```python
from build123d import *

# Parameters (mm, degrees)
F0_R     = 28.446673
F1_DEPTH = 25
F2_W     = 12.863994
F2_H     = 8.371785
F3_DEPTH = 25
F5_DEPTH = 25
F6_R     = 14.342599
F7_DEPTH = 125


with BuildPart() as f1:
    # F0 (on Front) → F1 (new body)
    with BuildSketch(Plane.XZ):
        Circle(F0_R)
    extrude(amount=F1_DEPTH)

    # F2 (on Front) → F3 (cut)
    with BuildSketch(Plane.XZ):
        with Locations((-6.431997, 4.185892)):
            Rectangle(F2_W, F2_H)
    extrude(amount=F3_DEPTH, mode=Mode.SUBTRACT)

    # F4 (on Front) → F5 (cut)
    with BuildSketch(Plane.XZ):
        Polygon((13.908368, -11.549142), (9.61332, 23.327414), (2.882242, 23.327414), (6.163642, -12.263194), align=None)
    extrude(amount=F5_DEPTH, mode=Mode.SUBTRACT)

    # F6 (on Front) → F7 (join)
    with BuildSketch(Plane.XZ):
        Circle(F6_R)
    extrude(amount=-F7_DEPTH)


solid = f1.part
```
Part model, mm, in its own coordinate system. A direction names the side the tool comes from. Round coordinates to 2 decimals unless told otherwise and drop trailing zeros. Write each loop counter-clockwise with the first axis right and the second up, starting at its lowest first coordinate (ties: lowest second). Pieces come first, ordered by that corner, then holes. Notation, with made-up numbers: (26.25, -24) -> (70.25, -24) arc R35 cw to (70.25, 14) -> close; hole circle Ø11 at (9, -22.5). An arc over 180 degrees is marked (long way). Return JSON: item names as keys, results as strings. Group by question number.
Q1. Saw through at B-B on y = 57. Write the cut outline in (x, z).
Q2. Probe L1, parallel to Y at x = 10, z = 2.5; L2, parallel to Y at x = -14.5, z = -7; L3, parallel to Z at x = -16, y = -16. List the from-to ranges inside material, lowest first. Write a range as [from, to].
Q3. Saw through at A-A on z = 21. Write the cut outline in (x, y).
Q4. Pin check, flat tips, straight feed: pin 1 (1.5 mm diameter, centred on x = -3.5, z = 19, fed in from +Y); pin 2 (12 mm diameter, centred on y = 39, z = -17.5, fed in from +X); pin 3 (2.5 mm diameter, centred on x = -8, z = 4.5, fed in from -Y). Stop position of each tip, or through.
Q5. Which spindle directions (+Z, -Z, +X, -X, +Y, -Y) get a long thin tool onto all of the face, cutting with end or side? Do faces 4 (the flat face through (6, -12, 23.327)), 5 (the flat face through (9.98, -12.32, -11.91)), 6 (the flat face through (0, 125, 0)), 7 (the flat face through (-13.04, 0, 6.72)). Say none if no direction does.
Q6. Mould opens along Z. For faces 1 (the flat face through (0, -12, 4)), 2 (the flat face through (0, -25, -6)), 3 (the cylindrical face through (13.68, 61.62, 4.31)) say: pulls with the +Z half, pulls with the -Z half, needs draft (parallel to the pull), parting line crosses it, or undercut.
Answer:
{
 "1": {"outline": "circle Ø28.69 at (0, 0)"},
 "2": {"L1": "[0, 125]", "L2": "[-25, 0]", "L3": "[-23.52, 23.52]"},
 "3": {"outline": "(-19.19, -25) -> (3.1, -25) -> (3.1, 0) -> (-19.19, 0) -> close; (9.9, -25) -> (19.19, -25) -> (19.19, 0) -> (9.9, 0) -> close"},
 "4": {"pin 1": "y = 0", "pin 2": "x = 8.57", "pin 3": "y = 0"},
 "5": {"face 4": "+Y, -Y", "face 5": "-Y", "face 6": "+Z, -Z, +X, -X, +Y", "face 7": "+Y"},
 "6": {"face 1": "undercut", "face 2": "needs draft", "face 3": "parting line crosses it"}
}
